Verification items for the finished model (mm, model axes). Face numbers are marked on the shaded views. A direction names the side the tool comes from. Coordinates: 2 decimals unless noted, no trailing zeros. Write each loop counter-clockwise with the first axis right and the second up, starting at its lowest first coordinate (ties: lowest second). Pieces come first, ordered by that corner, then holes. Notation, with made-up numbers: (12, 68) -> (46, 68) arc R14 ccw to (46, 75) -> close; hole circle Ø5 at (55, 85.25). An arc over 180 degrees is marked (long way). Write item = value, one per line. Start each with the question number.
(1) Mould release check, pull along Z, two halves, no side actions. Record for the marked faces 1, 2 and 3: released by +Z, released by -Z, zero draft, split by the parting line, or undercut.
(2) Section check C-C (x = 25). Record the cut outline in (y, z).
(3) Section check B-B (z = 16). Record the cut outline in (x, y), plus the area to 3 significant figures.
(4) Gauge pin test, flat end, axial feed: pin 1 Ø21.5 at (x, z) = (-6, -14.5) entering from -Y. Record the tip position at first contact, or that the pin passes through.
(5) Section check A-A (y = -449). Record the cut outline in (x, z), plus the area to 3 significant figures.
(6) Set-up check for the marked faces 4 and 5: record each of +Z, -Z, +X, -X, +Y, -Y from which the full face is reachable in a straight line by a thin tool's end or side.
(7) Material ranges on probe 1 along X at (y, z) = (-45.5, 28); probe 2 along Y at (x, z) = (22, -12.5), recorded low to high. Write a range as [from, to].
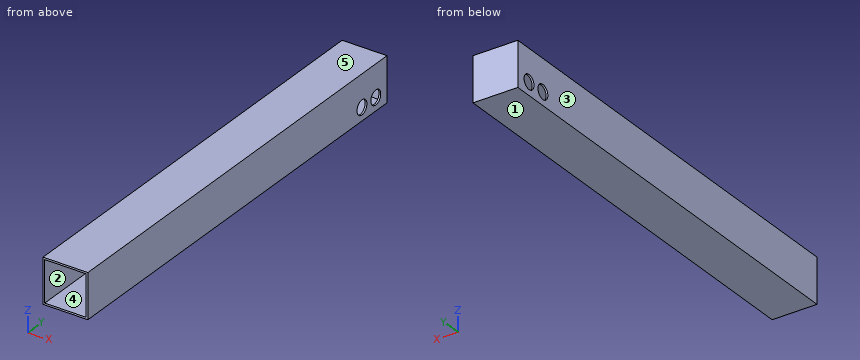
```python
from build123d import *

# Parameters (mm, degrees)
F0_W     = 77
F0_H     = 77
F1_DEPTH = 746
F2_T     = -3
F4_D     = 24.7
F6_D     = 24.7


with BuildPart() as f1:
    # F0 (on Front) → F1 (new body)
    with BuildSketch(Plane.XZ):
        Rectangle(F0_W, F0_H)
    extrude(amount=F1_DEPTH)

    # F2
    f2_openings = [f1.faces().sort_by_distance(p)[0] for p in [
        (0, -746, 0),
    ]]
    offset(amount=F2_T, openings=f2_openings)

    # F4 (through all)
    with Locations(Plane(origin=(-38.5, 0, 0), x_dir=(0, -1, 0), z_dir=(-1, 0, 0))):
        with Locations((27.953846, -16.379451)):
            Hole(F4_D / 2)

    # F6 (through all)
    with Locations(Plane(origin=(-38.5, 0, 0), x_dir=(0, -1, 0), z_dir=(-1, 0, 0))):
        with Locations((62.507309, -16.257038)):
            Hole(F6_D / 2)


solid = f1.part
```
Response:
q1.face_1 = released by -Z
q1.face_2 = undercut
q1.face_3 = zero draft
q2.outline = (-746, -38.5) -> (0, -38.5) -> (0, 38.5) -> (-746, 38.5) -> (-746, 35.5) -> (-3, 35.5) -> (-3, -35.5) -> (-746, -35.5) -> close
q3.outline = (-38.5, -746) -> (-35.5, -746) -> (-35.5, -3) -> (35.5, -3) -> (35.5, -746) -> (38.5, -746) -> (38.5, 0) -> (-38.5, 0) -> close
q3.area = 4,690 mm2
q4.pin_1 = -3
q5.outline = (-38.5, -38.5) -> (38.5, -38.5) -> (38.5, 38.5) -> (-38.5, 38.5) -> close; hole (-35.5, -35.5) -> (35.5, -35.5) -> (35.5, 35.5) -> (-35.5, 35.5) -> close
q5.area = 888 mm2
q6.face_4 = -Y
q6.face_5 = +Z, +X, -X, +Y, -Y
q7.probe_1 = [-38.5, -35.5], [35.5, 38.5]
q7.probe_2 = [-3, 0]
